Here's how the part is built. I have some questions about the finished solid (model axes, mm). Face numbers are marked on the shaded views. A direction names the side the tool comes from. Round coordinates to 2 decimals unless told otherwise and drop trailing zeros. Order: outer loops, then holes, each group sorted by start corner. A loop starts at its lowest first (then second) coordinate and runs counter-clockwise, first axis right, second up. Notation, with made-up numbers: (-17, -25) -> (42, -25) arc R19 cw to (42, -20) -> close; hole circle Ø4 at (44, 17.25). An arc over 180 degrees is marked (long way). Answer in a Markdown table with one row per item.
```python
from build123d import *

# Parameters (mm, degrees)
F0_W     = 18.5
F0_H     = 13
F1_DEPTH = 10
F0_W_2   = 3
F0_H_2   = 2.95
F2_DEPTH = 14
F4_DEPTH = 7
F5_R     = 4
F5_R_2   = 2.25
F6_DEPTH = 6


# Not quite as in the source:
# - a fillet or chamfer that OpenCascade refuses, or shapes differently, is made with other operations: its cross-section is extruded or revolved along the edge and cut away or added


with BuildPart() as f1:
    # F0 (on Top) → F1 (new body)
    with BuildSketch(Plane.XY):
        with BuildLine():
            Line((-4.96357069, 33), (-4.96357069, 25.95))
            Line((-4.96357069, 25.95), (-1.96357069, 25.95))
            Line((-1.96357069, 25.95), (-1.96357069, 23))
            Line((-1.96357069, 23), (2.03642931, 23))
            ThreePointArc((2.03642931, 23), (4.28642931, 25.25), (6.53642931, 23))
            Line((6.53642931, 23), (10.53642931, 23))
            Line((10.53642931, 23), (10.53642931, 25.95))
            Line((10.53642931, 25.95), (13.53642931, 25.95))
            Line((13.53642931, 25.95), (13.53642931, 33))
            Line((13.53642931, 33), (-4.96357069, 33))
        make_face()
        with BuildLine():
            Line((-4.96357069, 20.05), (-4.96357069, 13))
            Line((-4.96357069, 13), (13.53642931, 13))
            Line((13.53642931, 13), (13.53642931, 20.05))
            Line((13.53642931, 20.05), (10.53642931, 20.05))
            Line((10.53642931, 20.05), (10.53642931, 23))
            Line((10.53642931, 23), (6.53642931, 23))
            ThreePointArc((6.53642931, 23), (4.28642931, 20.75), (2.03642931, 23))
            Line((2.03642931, 23), (-1.96357069, 23))
            Line((-1.96357069, 23), (-1.96357069, 20.05))
            Line((-1.96357069, 20.05), (-4.96357069, 20.05))
        make_face()
        with Locations((4.28642931, 6.5)):
            Rectangle(F0_W, F0_H)
    extrude(amount=F1_DEPTH)

    # F0 (on Top) → F2 (join)
    with BuildSketch(Plane.XY):
        with Locations((-3.46357069, 21.525)):
            Rectangle(F0_W_2, F0_H_2)
        with Locations((-3.46357069, 24.475)):
            Rectangle(F0_W_2, F0_H_2)
        with Locations((12.03642931, 24.475)):
            Rectangle(F0_W_2, F0_H_2)
        with Locations((12.03642931, 21.525)):
            Rectangle(F0_W_2, F0_H_2)
    extrude(amount=F2_DEPTH)

    # F3 (on face) → F4 (cut)
    with BuildSketch(Plane.XZ):
        Polygon((3.8593590405, 10), (1.9593590405, 10), (1.9593590405, 9), (2.9593590405, 9), (2.9593590405, 8), (1.9593590405, 8), (1.9593590405, 7), (2.9593590405, 7), (2.9593590405, 6), (1.9593590405, 6), (1.9593590405, 5), (2.9593590405, 5), (2.9593590405, 4), (1.9593590405, 4), (1.9593590405, 3), (2.9593590405, 3), (2.9593590405, 2), (1.9593590405, 2), (1.9593590405, 1), (2.9593590405, 1), (2.9593590405, 0), (3.8593590405, 0), align=None)
    extrude(amount=-F4_DEPTH, mode=Mode.SUBTRACT)

    # F5 (on face) → F6 (cut)
    with BuildSketch(Plane(origin=(0, 0, 0), x_dir=(1, 0, 0), z_dir=(0, 0, -1))):
        with Locations((4.28642931, -23)):
            Circle(F5_R)
        with Locations((4.28642931, -23)):
            Circle(F5_R_2, mode=Mode.SUBTRACT)
    extrude(amount=-F6_DEPTH, mode=Mode.SUBTRACT)

    # F7: fillet of radius 3 on 1 edges, made by hand

    # F7_s1 → F7_t2 (revolve)
    with BuildSketch(Plane.XZ.offset(-23)):
        with BuildLine():
            ThreePointArc((8.28642931, 3.2728219713), (7.8113055446, 4.8930071459), (6.53642931, 6))
            Line((6.53642931, 6), (8.28642931, 6))
            Line((8.28642931, 6), (8.28642931, 3.2728219713))
        make_face()
    revolve(axis=Axis((4.28642931, 23, 6), (0, 0, -1)))


solid = f1.part
```
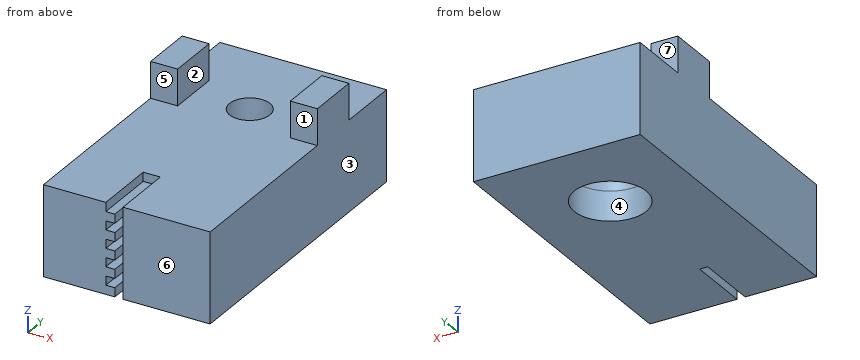
1. Suppose I cut it at C-C on x = -3. Write out the boundary of the cut face in (y, z), then the cut area to 3 significant figures.
Numbers:
| item | result |
|---|---|
| outline | (0, 0) -> (33, 0) -> (33, 10) -> (25.95, 10) -> (25.95, 14) -> (20.05, 14) -> (20.05, 10) -> (0, 10) -> close |
| area | 354 mm2 |
2. Suppose I cut it at B-B on y = 5. Write out the boundary of the cut face in (x, z).
Numbers:
| item | result |
|---|---|
| outline | (-4.96, 0) -> (2.96, 0) -> (2.96, 1) -> (1.96, 1) -> (1.96, 2) -> (2.96, 2) -> (2.96, 3) -> (1.96, 3) -> (1.96, 4) -> (2.96, 4) -> (2.96, 5) -> (1.96, 5) -> (1.96, 6) -> (2.96, 6) -> (2.96, 7) -> (1.96, 7) -> (1.96, 8) -> (2.96, 8) -> (2.96, 9) -> (1.96, 9) -> (1.96, 10) -> (-4.96, 10) -> close; (3.86, 0) -> (13.54, 0) -> (13.54, 10) -> (3.86, 10) -> close |
3. We'd pull the mould along X, two halves only. Please class the marked faces 1, 2 and 3: released by +X, released by -X, zero draft, split by the parting line, or undercut.
Numbers:
| item | result |
|---|---|
| face 1 | zero draft |
| face 2 | undercut |
| face 3 | released by +X |
4. For pin 1 Ø2 at (y, z) = (11, 12) entering from +X; pin 2 Ø2 at (x, y) = (-0.5, 15) entering from -Z; pin 3 Ø0.5 at (x, y) = (2, 4.5) entering from +Z; pin 4 Ø0.5 at (x, y) = (2.5, 3.5) entering from +Z, each with a flat end and sliding along its axis, tell me the tip position at first contact or that it passes through.
Numbers:
| item | result |
|---|---|
| pin 1 | passes through |
| pin 2 | stops at z = 0 |
| pin 3 | stops at z = 10 |
| pin 4 | stops at z = 9 |
5. Suppose I cut it at A-A on z = 10.5. Write out the boundary of the cut face in (x, y), then the cut area to 3 significant figures.
Numbers:
| item | result |
|---|---|
| outline | (-4.96, 20.05) -> (-1.96, 20.05) -> (-1.96, 25.95) -> (-4.96, 25.95) -> close; (10.54, 20.05) -> (13.54, 20.05) -> (13.54, 25.95) -> (10.54, 25.95) -> close |
| area | 35.4 mm2 |
6. Please list where these lines run through material, in increasing order: line 1 along X through (y, z) = (23, 9.15); line 2 along X through (y, z) = (3, 6.25); line 3 along Z through (x, y) = (8, 16).
Numbers:
| item | result |
|---|---|
| line 1 | x = -4.96 to 2.04, 6.54 to 13.54 |
| line 2 | x = -4.96 to 2.96, 3.86 to 13.54 |
| line 3 | z = 0 to 10 |
7. For the marked faces 4, 5, 6 and 7, which set-ups out of +Z, -Z, +X, -X, +Y, -Y let a thin tool reach every point of the face, with its end or its side?
Numbers:
| item | result |
|---|---|
| face 4 | -Z |
| face 5 | +Z, +X, -X, -Y |
| face 6 | +Z, -Z, +X, -X, -Y |
| face 7 | +Z, +X, -X, +Y |
